Read the model definition and answer for the solid it produces. Units are mm, in the model's axes. A direction names the side the tool comes from. Give positions to 0.01 mm unless a question says otherwise; leave off trailing zeros. Order: outer loops, then holes, each group sorted by start corner. A loop starts at its lowest first (then second) coordinate and runs counter-clockwise, first axis right, second up. Notation, with made-up numbers: (59.25, 19.25) -> (117.25, 19.25) arc R22 ccw to (117.25, 58.25) -> close; hole circle Ø7 at (-12, 7.5). An arc over 180 degrees is marked (long way). One line per item, written item: value. Start each with the question number.
from build123d import *

# Parameters (mm, degrees)
SKETCH1_R           = 87.5
BOSS_EXTRUDE1_DEPTH = 20
SKETCH2_R           = 25
CUT_EXTRUDE1_DEPTH  = 126.349511367
SKETCH3_R           = 10
CUT_EXTRUDE2_DEPTH  = 18.298379
CIRPATTERN1_START   = 1.701620914
CIRPATTERN1_DEPTH   = 18.298379086


# Read off the part's stored shape, not the designer's step: CirPattern1
with BuildPart() as part:
    # Sketch1 → Boss-Extrude1 (new body)
    with BuildSketch(Plane(origin=(0, 0, 0), x_dir=(1, 0, 0), z_dir=(0, 1, 0))):
        with Locations(Location((0, 0, 0), (0, 0, 270))):
            Circle(SKETCH1_R)
    extrude(amount=BOSS_EXTRUDE1_DEPTH)

    # Sketch2 → Cut-Extrude1 (cut, through all)
    with BuildSketch(Plane(origin=(0, 0, 0), x_dir=(1, 0, 0), z_dir=(0, 1, 0))):
        with Locations(Location((0, 0, 0), (0, 0, 270))):
            Circle(SKETCH2_R)
    extrude(amount=CUT_EXTRUDE1_DEPTH, mode=Mode.SUBTRACT)

    # Sketch3 → Cut-Extrude2 (cut)
    with BuildSketch(Plane(origin=(0, 20, 0), x_dir=(1, 0, 0), z_dir=(0, 1, 0))):
        with Locations((-29.38501669, 0)):
            Circle(SKETCH3_R)
    extrude(amount=-CUT_EXTRUDE2_DEPTH, mode=Mode.SUBTRACT)

    # CirPattern1 outline → CirPattern1 (cut)
    with BuildSketch(Plane(origin=(0, 0, 0), x_dir=(1, 0, 0), z_dir=(0, 1, 0)).offset(CIRPATTERN1_START)):
        with BuildLine():
            ThreePointArc((-4.733118503, -24.547863232), (-12.5, -21.650635094), (-18.892513916, -16.372932478))
            ThreePointArc((-18.892513916, -16.372932478), (-19.692508346, -34.108424982), (-4.733118503, -24.547863232))
        make_face()
        with BuildLine():
            ThreePointArc((-4.733118503, 24.547863232), (-19.692508346, 34.108424982), (-18.892513916, 16.372932478))
            ThreePointArc((-18.892513916, 16.372932478), (-12.5, 21.650635094), (-4.733118503, 24.547863232))
        make_face()
        with BuildLine():
            ThreePointArc((18.892513916, -16.372932478), (12.5, -21.650635094), (4.733118503, -24.547863232))
            ThreePointArc((4.733118503, -24.547863232), (19.692508346, -34.108424982), (18.892513916, -16.372932478))
        make_face()
        with BuildLine():
            ThreePointArc((18.892513916, 16.372932478), (19.692508346, 34.108424982), (4.733118503, 24.547863232))
            ThreePointArc((4.733118503, 24.547863232), (12.5, 21.650635094), (18.892513916, 16.372932478))
        make_face()
        with BuildLine():
            ThreePointArc((23.625632419, 8.174930753), (25, 0), (23.625632419, -8.174930753))
            ThreePointArc((23.625632419, -8.174930753), (39.38501669, 0), (23.625632419, 8.174930753))
        make_face()
    extrude(amount=CIRPATTERN1_DEPTH, mode=Mode.SUBTRACT)


solid = part.part
Item 1: Find section B-B on x = 0. Write down the section's boundary in (y, z), then the cut area to 3 significant figures.
Item 2: Find the intervals of material crossed by line 1 (X direction, y = 1.5, z = 0.5) (3 decimals); line 2 (Z direction, x = 34, y = 5.75); line 3 (X direction, y = 6.5, z = 30), in increasing order. Write a range as from..to.
Item 3: Find section D-D on z = -32. Write down the section's boundary in (x, y), then the cut area to 3 significant figures.
Item 4: For a pull along Z with two mould halves and no side action, classify faces 1 (the cylindrical face through (-39.38, 10.98, -0.31)), 2 (the flat face through (-18, 0, 18)), 3 (the cylindrical face through (86.755, 9.86, -11.391)) as +Z half, -Z half, draft (parallel to the pull), parting line (faces both ways), or undercut.
Item 5: Find section A-A on z = 0. Write down the section's boundary in (x, y).
Item 6: Flat-ended cylindrical pins translate along their axes: pin 1 (5.5 mm diameter, centred on x = 17, z = 25, fed in from +Y); pin 2 (10 mm diameter, centred on y = 9.5, z = 48, fed in from -X); pin 3 (2 mm diameter, centred on y = 8.5, z = -55, fed in from -X). Find the tip coordinate at first contact, or state that the pin passes through.
Item 7: A tool of negligible diameter and unlimited length cuts with its end or side. For faces 4 (the cylindrical face through (19.955, 10.723, -33.951)), 5 (the cylindrical face through (-22.2, 7.6, 11.5)), from which of +Z, -Z, +X, -X, +Y, -Y can it reach the whole face along a straight path? Write none if from no direction.
Item 8: Find section C-C on y = 16. Write down the section's boundary in (x, z), then the cut area to 3 significant figures.
Checks:
1. outline: (0, -87.5) -> (20, -87.5) -> (20, -25) -> (0, -25) -> close; (0, 25) -> (20, 25) -> (20, 87.5) -> (0, 87.5) -> close
1. area: 2,500 mm2
2. line 1: -87.499..-24.995, 24.995..87.499
2. line 2: -80.62..-8.87, 8.87..80.62
2. line 3: -82.2..-23.6, -5.79..5.79, 23.6..82.2
3. outline: (-81.44, 0) -> (81.44, 0) -> (81.44, 20) -> (22.25, 20) -> (22.25, 1.7) -> (7.14, 1.7) -> (7.14, 20) -> (-7.14, 20) -> (-7.14, 1.7) -> (-22.25, 1.7) -> (-22.25, 20) -> (-81.44, 20) -> close
3. area: 2,700 mm2
4. face 1: undercut
4. face 2: draft
4. face 3: parting line
5. outline: (-87.5, 0) -> (-25, 0) -> (-25, 1.7) -> (-39.39, 1.7) -> (-39.39, 20) -> (-87.5, 20) -> close; (25, 0) -> (87.5, 0) -> (87.5, 20) -> (39.39, 20) -> (39.39, 1.7) -> (25, 1.7) -> close
6. pin 1: y = 1.7
6. pin 2: x = -76.21
6. pin 3: x = -68.85
7. face 4: +Y
7. face 5: +Y, -Y
8. outline: circle Ø175 at (0, 0); hole (-23.63, -8.17) arc R25 ccw to (-18.89, -16.37) arc R10 ccw (long way) to (-4.73, -24.55) arc R25 ccw to (4.73, -24.55) arc R10 ccw (long way) to (18.89, -16.37) arc R25 ccw to (23.63, -8.17) arc R10 ccw (long way) to (23.63, 8.17) arc R25 ccw to (18.89, 16.37) arc R10 ccw (long way) to (4.73, 24.55) arc R25 ccw to (-4.73, 24.55) arc R10 ccw (long way) to (-18.89, 16.37) arc R25 ccw to (-23.63, 8.17) arc R10 ccw (long way) to start
8. area: 20,600 mm2
